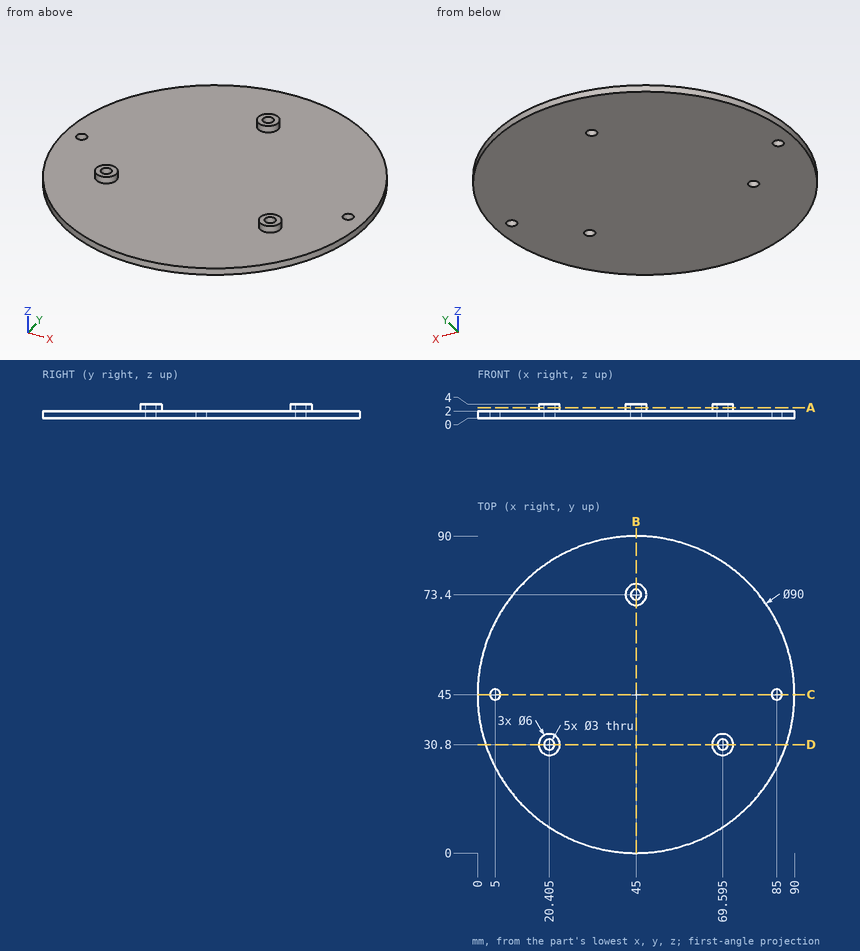
Source: three-view drawing plus pictorial views. Frame: mm from the lowest corner of the part. Coordinates: 2 decimals unless noted, no trailing zeros. Loops run counter-clockwise (first coordinate to the right, second up) from the corner with the lowest first, then second, coordinate; pieces in that order, holes last. Notation, with made-up numbers: (-30, 5.25) -> (8, 5.25) arc R23 ccw to (8, 32.25) -> close; hole circle Ø3 at (-30, 0.25). An arc over 180 degrees is marked (long way). Answer in a Markdown table with one row per item. Add a question column.
Q1. Ray query, line 1 along X through (y, z) = (73.4, 3.15); line 2 along Z through (x, y) = (45, 42); line 3 along Y through (x, z) = (5, 1.25) (1 decimal). Return the intervals inside material, ascending.
Q2. Contact query for a flat-ended pin moving along its axis: pin 1 Ø1 at (x, y) = (46.5, 37.5) entering from +Z. Output: stop coordinate, or through.
Q3. Section C-C on y = 45. Return the cut outline in (x, z).
Q4. Section B-B on x = 45. Return the cut outline in (y, z).
Q5. Section D-D on y = 30.8. Return the cut outline in (x, z) (3 decimals), and give its area (3 significant figures).
Q6. Section A-A on z = 2.95. Return the cut outline in (x, y) (3 decimals).
Computed values:
| question | item | result |
|---|---|---|
| 1 | line 1 | x = 42 to 43.5, 46.5 to 48 |
| 1 | line 2 | z = 0 to 2 |
| 1 | line 3 | y = 24.4 to 43.5, 46.5 to 65.6 |
| 2 | pin 1 | stops at z = 2 |
| 3 | outline | (0, 0) -> (3.5, 0) -> (3.5, 2) -> (0, 2) -> close; (6.5, 0) -> (83.5, 0) -> (83.5, 2) -> (6.5, 2) -> close; (86.5, 0) -> (90, 0) -> (90, 2) -> (86.5, 2) -> close |
| 4 | outline | (0, 0) -> (71.9, 0) -> (71.9, 4) -> (70.4, 4) -> (70.4, 2) -> (0, 2) -> close; (74.9, 0) -> (90, 0) -> (90, 2) -> (76.4, 2) -> (76.4, 4) -> (74.9, 4) -> close |
| 5 | outline | (2.299, 0) -> (18.905, 0) -> (18.905, 4) -> (17.405, 4) -> (17.405, 2) -> (2.299, 2) -> close; (21.905, 0) -> (68.095, 0) -> (68.095, 4) -> (66.595, 4) -> (66.595, 2) -> (23.405, 2) -> (23.405, 4) -> (21.905, 4) -> close; (71.095, 0) -> (87.701, 0) -> (87.701, 2) -> (72.595, 2) -> (72.595, 4) -> (71.095, 4) -> close |
| 5 | area | 171 mm^2 |
| 6 | outline | circle Ø6 at (20.405, 30.8); circle Ø6 at (45, 73.4); circle Ø6 at (69.595, 30.8); hole circle Ø3 at (20.405, 30.8); hole circle Ø3 at (45, 73.4); hole circle Ø3 at (69.595, 30.8) |
